CAD build for the part. Positions are in the model's coordinates, mm. A direction names the side the tool comes from. Coordinates: 2 decimals unless noted, no trailing zeros. Write each loop counter-clockwise with the first axis right and the second up, starting at its lowest first coordinate (ties: lowest second). Pieces come first, ordered by that corner, then holes. Notation, with made-up numbers: (13.25, -14) -> (58.25, -14) arc R33 cw to (58.25, 20) -> close; hole circle Ø10 at (23.25, 19). An arc over 180 degrees is marked (long way). Answer as CSV lines item,"result".
```python
from build123d import *

# Parameters (mm, degrees)
SKETCH1_R           = 1
BOSS_EXTRUDE4_DEPTH = 1
SKETCH4_R           = 1
BOSS_EXTRUDE5_DEPTH = 1


with BuildPart() as part:
    # Sketch1 → Boss-Extrude4 (new body)
    with BuildSketch(Plane(origin=(0, 0, 0), x_dir=(1, 0, 0), z_dir=(0, 1, 0))):
        with BuildLine():
            Line((-26.085, 3), (23.915, 3))
            ThreePointArc((23.915, 3), (27.965705649, 2.046261886), (28.743665769, -2.041844117))
            Line((28.743665769, -2.041844117), (20.812640503, -15.067570319))
            ThreePointArc((20.812640503, -15.067570319), (19.103092744, -15.647684769), (17.322461075, -15.350300892))
            Line((17.322461075, -15.350300892), (-26.085, -3))
            ThreePointArc((-26.085, -3), (-29.085, 0), (-26.085, 3))
        make_face()
        with Locations((-26.085, 0)):
            Circle(SKETCH1_R, mode=Mode.SUBTRACT)
        with Locations((26.085, 0)):
            Circle(SKETCH1_R, mode=Mode.SUBTRACT)
    extrude(amount=BOSS_EXTRUDE4_DEPTH)

    # Sketch4 → Boss-Extrude5 (add)
    with BuildSketch(Plane(origin=(0, 1, 0), x_dir=(1, 0, 0), z_dir=(0, 1, 0))):
        with Locations((17.732709605, -11.715326645)):
            Circle(SKETCH4_R)
    extrude(amount=BOSS_EXTRUDE5_DEPTH)


solid = part.part
```
Item 1: Saw through at A-A on z = -0.5. Give the cut face in (x, y).
Answer below:
outline,"(-29.04, 0) -> (-26.95, 0) -> (-26.95, 1) -> (-29.04, 1) -> close; (-25.22, 0) -> (25.22, 0) -> (25.22, 1) -> (-25.22, 1) -> close; (26.95, 0) -> (28.87, 0) -> (28.87, 1) -> (26.95, 1) -> close"
Item 2: Saw through at C-C on z = 10. Give the cut face in (x, y), and give its area (3 significant figures).
Answer below:
outline,"(-1.48, 0) -> (23.9, 0) -> (23.9, 1) -> (-1.48, 1) -> close"
area,"25.4 mm2"
Item 3: Saw through at B-B on x = -22. Give the cut face in (y, z), and give its area (3 significant figures).
Answer below:
outline,"(0, -3) -> (1, -3) -> (1, 4.16) -> (0, 4.16) -> close"
area,"7.16 mm2"
Item 4: Wall check: line 1 (X direction, y = 0.4, z = 0) (3 decimals); line 2 (Z direction, x = 26.5, y = 0.7); line 3 (Y direction, x = 12.5, z = 4). Give the ranges that are in metal, low to high. Write a range as from..to.
Answer below:
line 1,"x = -29.085..-27.085, -25.085..25.085, 27.085..28.98"
line 2,"z = -3..-0.91, 0.91..5.73"
line 3,"y = 0..1"
Item 5: Flat gauge pins, fed straight in: pin 1 (10 mm diameter, centred on x = -18.5, z = -1, fed in from +Y); pin 2 (1.5 mm diameter, centred on x = 13, z = 5.5, fed in from -Y); pin 3 (0.8 mm diameter, centred on x = 11, y = 0.5, fed in from -Z). Where does each tip first touch, or does it go through?
Answer below:
pin 1,"stops at y = 1"
pin 2,"stops at y = 0"
pin 3,"stops at z = -3"
Item 6: 3-axis set-ups, long thin cutter, end or side, ignore diameter. For faces 5 (the flat face through (-1.4, 0.5, -3)), 6 (the cylindrical face through (19.129, 0.493, 15.646)): which of +Z, -Z, +X, -X, +Y, -Y reach the whole face in a straight line?
Answer below:
face 5,"-Z, -X, +Y, -Y"
face 6,"+Z, +Y, -Y"
Item 7: Saw through at D-D on y = 1.3. Give the cut face in (x, z), and give its area (3 significant figures).
Answer below:
outline,"circle Ø2 at (17.73, 11.72)"
area,"3.14 mm2"
Item 8: Two-plate mould, pull along X, no slides. Class faces 1 (the cylindrical face through (16.939, 1.493, 12.324)), 2 (the cylindrical face through (27, 0.5, 0.4)), 3 (the flat face through (-4.08, 0.49, 9.26)), 4 (the cylindrical face through (-25.16, 0.49, 0.38)): pulls with the +X half, pulls with the -X half, needs draft (parallel to the pull), parting line crosses it, or undercut.
Answer below:
face 1,"parting line crosses it"
face 2,"undercut"
face 3,"pulls with the -X half"
face 4,"undercut"
